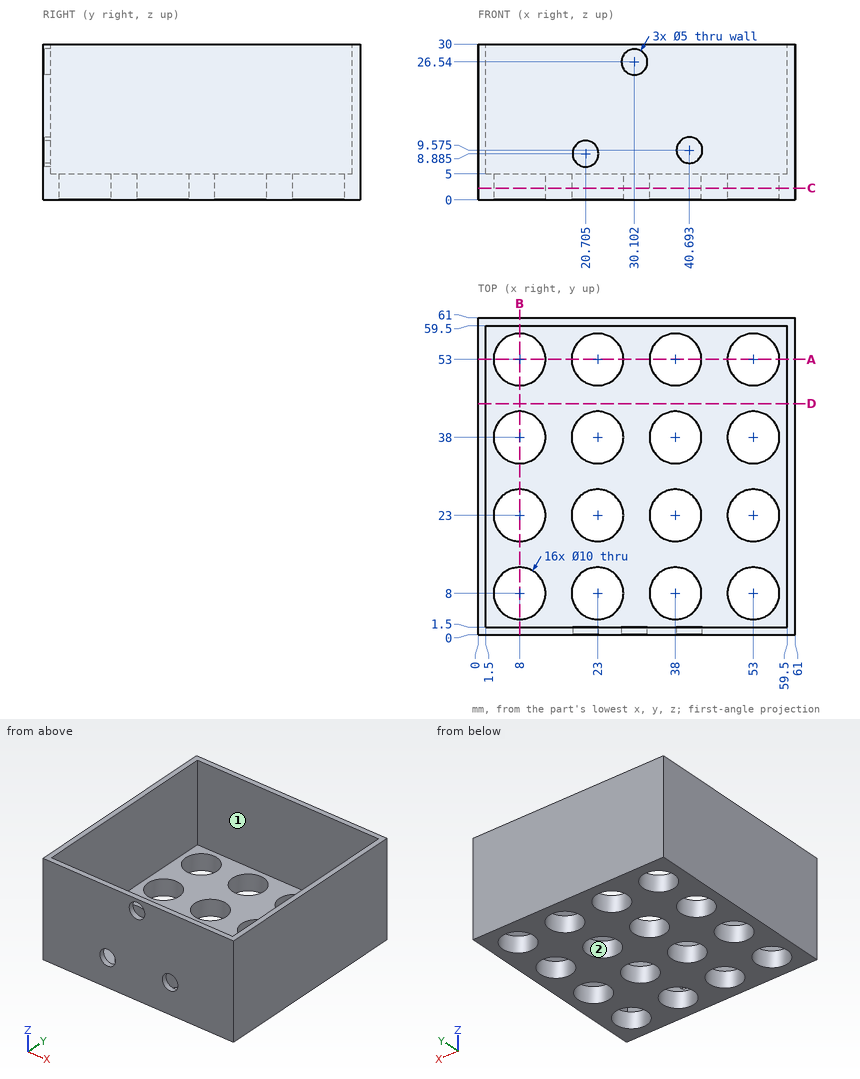
For this review, use the dimensioned drawing (mm, ordinates from the lowest corner) and the shaded views. A direction names the side the tool comes from. Coordinates: 2 decimals unless noted, no trailing zeros. Write each loop counter-clockwise with the first axis right and the second up, starting at its lowest first coordinate (ties: lowest second). Pieces come first, ordered by that corner, then holes. Notation, with made-up numbers: (-13.5, -5) -> (21.5, -5) arc R26 cw to (21.5, 20) -> close; hole circle Ø9 at (-22, 67). An arc over 180 degrees is marked (long way). Put each result on its own line as item: value.
Q1. Take a section at C-C, the plane z = 2.25. Count the separate pieces of the cut face and the enclosed holes in it, then the cut area to 3 significant figures.
From the geometry:
separate pieces: 1
enclosed holes: 16
area: 2,460 mm2
Q2. Tool access review of the marked faces 1 and 2: name each direction out of +Z, -Z, +X, -X, +Y, -Y from which nothing blocks a thin tool from reaching the whole face with its end or side.
From the geometry:
face 1: +Z
face 2: +Z, -Z
Q3. Take a section at A-A, the plane y = 53. State the section outline as (x, z) points.
From the geometry:
outline: (0, 0) -> (3, 0) -> (3, 5) -> (1.5, 5) -> (1.5, 30) -> (0, 30) -> close; (13, 0) -> (18, 0) -> (18, 5) -> (13, 5) -> close; (28, 0) -> (33, 0) -> (33, 5) -> (28, 5) -> close; (43, 0) -> (48, 0) -> (48, 5) -> (43, 5) -> close; (58, 0) -> (61, 0) -> (61, 30) -> (59.5, 30) -> (59.5, 5) -> (58, 5) -> close
Q4. Clearance check with flat-ended pins moving along their axes: pin 1 Ø4 at (x, y) = (51.5, 44) entering from -Z; pin 2 Ø1 at (x, y) = (47.5, 26.5) entering from +Z. State where each tip first meets the part, or that it passes through.
From the geometry:
pin 1: stops at z = 0
pin 2: stops at z = 5
Q5. Take a section at D-D, the plane y = 44.5. State the section outline as (x, z) points.
From the geometry:
outline: (0, 0) -> (61, 0) -> (61, 30) -> (59.5, 30) -> (59.5, 5) -> (1.5, 5) -> (1.5, 30) -> (0, 30) -> close
Q6. Wall thickness on L1, parallel to Y at x = 53, z = 3; L2, parallel to Y at x = 11, z = 16.5: over which ranges is each line inside the solid? List them lowest first.
From the geometry:
L1: y = 0 to 3, 13 to 18, 28 to 33, 43 to 48, 58 to 61
L2: y = 0 to 1.5, 59.5 to 61
